Part model, mm, in its own coordinate system. A direction names the side the tool comes from. Coordinates: 2 decimals unless noted, no trailing zeros. Order: outer loops, then holes, each group sorted by start corner. A loop starts at its lowest first (then second) coordinate and runs counter-clockwise, first axis right, second up.
```python
from build123d import *
from build123d.topology import SkipClean

# Parameters (mm, degrees)
CROQUIS1_R                                           = 11.75
SALIENTE_EXTRUIR1_DEPTH                              = 5
REFRENTADO_PARA_TORNILLO_CON_CABEZA_PLAN_D           = 2
REFRENTADO_PARA_TORNILLO_CON_CABEZA_PLAN_CBORE_D     = 4
REFRENTADO_PARA_TORNILLO_CON_CABEZA_PLAN_CBORE_DEPTH = 2.5
CROQUIS6_R                                           = 4.25
CORTAR_EXTRUIR1_DEPTH                                = 1.9
CROQUIS7_R                                           = 5.75
SALIENTE_EXTRUIR2_DEPTH                              = 15
CROQUIS8_R                                           = 5.75
SALIENTE_EXTRUIR3_DEPTH                              = 10
CROQUIS9_R                                           = 3.55
CORTAR_EXTRUIR2_DEPTH                                = 20
SALIENTE_EXTRUIR4_DEPTH                              = 10
CORTAR_EXTRUIR3_DEPTH                                = 3
MATRIZC1_COUNT                                       = 4


with BuildPart() as part:
    # Croquis1 → Saliente-Extruir1 (new body)
    with BuildSketch(Plane.XY):
        Circle(CROQUIS1_R)
    extrude(amount=SALIENTE_EXTRUIR1_DEPTH)

    # Refrentado para tornillo con cabeza plana de M21 (through all)
    with Locations(Plane(origin=(0, 8, 5), x_dir=(1, 0, 0), z_dir=(0, 0, 1))):
        with Locations((0, 0), (7.999986777, -7.985454569), (0, -16), (-8, -8)):
            CounterBoreHole(REFRENTADO_PARA_TORNILLO_CON_CABEZA_PLAN_D / 2, REFRENTADO_PARA_TORNILLO_CON_CABEZA_PLAN_CBORE_D / 2, REFRENTADO_PARA_TORNILLO_CON_CABEZA_PLAN_CBORE_DEPTH)

    # Croquis6 → Cortar-Extruir1 (cut)
    with BuildSketch(Plane(origin=(0, 0, 0), x_dir=(-1, 0, 0), z_dir=(0, 0, -1))):
        with Locations((0, 0.014473443)):
            Circle(CROQUIS6_R)
    extrude(amount=-CORTAR_EXTRUIR1_DEPTH, mode=Mode.SUBTRACT)

    # Croquis7 → Saliente-Extruir2 (add)
    with BuildSketch(Plane.XY.offset(5)):
        Circle(CROQUIS7_R)
    extrude(amount=SALIENTE_EXTRUIR2_DEPTH)

    # Croquis8 → Saliente-Extruir3 (add)
    with BuildSketch(Plane.XY.offset(20)):
        Circle(CROQUIS8_R)
    extrude(amount=SALIENTE_EXTRUIR3_DEPTH)

    # Croquis9 → Cortar-Extruir2 (cut)
    with BuildSketch(Plane.XY.offset(30)):
        Circle(CROQUIS9_R)
    extrude(amount=-CORTAR_EXTRUIR2_DEPTH, mode=Mode.SUBTRACT)

    # Croquis10 → Saliente-Extruir4 (add)
    with SkipClean():  # the faces are left unmerged after this step: merging them gives an invalid solid
        with BuildSketch(Plane.XY.offset(5)):
            with BuildLine():
                Line((-7.342883246, 5.221562902), (-9.301185034, 7.17986469))
                ThreePointArc((-9.301185034, 7.17986469), (-8.308504679, 8.308504679), (-7.17986469, 9.301185034))
                Line((-7.17986469, 9.301185034), (-5.221562902, 7.342883246))
                Line((-5.221562902, 7.342883246), (-2.864419445, 4.985739789))
                ThreePointArc((-2.864419445, 4.985739789), (-4.065863992, 4.065863992), (-4.985739789, 2.864419445))
                Line((-4.985739789, 2.864419445), (-7.342883246, 5.221562902))
            make_face()
        saliente_extruir4 = extrude(amount=SALIENTE_EXTRUIR4_DEPTH)

    # Croquis11 → Cortar-Extruir3 (cut)
    with BuildSketch(Plane(origin=(-1.060660172, -1.060660172, 0), x_dir=(0, 0, 1), z_dir=(-0.7071067811865472, -0.7071067811865478, 0))):
        Polygon((15, 5.550900828), (15, 11.784165538), (5, 11.780723295), (5, 11.653862021), align=None)
    cortar_extruir3 = extrude(amount=-CORTAR_EXTRUIR3_DEPTH, mode=Mode.SUBTRACT)

    # MatrizC1: Saliente-Extruir4, Cortar-Extruir3 ×4 about axis
    with SkipClean():  # the faces are left unmerged after this step: merging them gives an invalid solid
        matrizc1_axis = Axis((0, 0, 0), (0, 0, 1))
        add([saliente_extruir4.rotate(matrizc1_axis, i * 360 / MATRIZC1_COUNT) for i in range(1, MATRIZC1_COUNT)])
        add([cortar_extruir3.rotate(matrizc1_axis, i * 360 / MATRIZC1_COUNT) for i in range(1, MATRIZC1_COUNT)], mode=Mode.SUBTRACT)


solid = part.part
```
(1) Drop flat-ended pins along their axis: pin 1 (4 mm diameter, centred on x = -7, y = -9, fed in from +Z); pin 2 (3 mm diameter, centred on x = -9, y = -1, fed in from +Z); pin 3 (4 mm diameter, centred on y = 9, z = 4.5, fed in from +X). Give the stop position or say it passes through.
(2) Slice it at C-C, the plane z = 10.5. Give the cut face in (x, y).
(3) Slice it at A-A, the plane x = 0. State how many separate pieces and enclosed holes the cut face has, then the cut area to 3 significant figures.
(4) Probe line 1 (Y direction, x = 0, z = 1.3); line 2 (Y direction, x = 0, z = 4.1); line 3 (Y direction, x = -0.5, z = 3.5). List the from-to ranges inside material, lowest first.
(5) Slice it at B-B, the plane y = 8. Give the cut face in (x, z).
(6) Tool access for faces 1 (the face through (-6.21, 4.09, 7.71)), 2 (the face through (6, 0, 4)), 3 (the face through (4.51, -6.63, 8.82)): list every direction of +Z, -Z, +X, -X, +Y, -Y with a clear straight run to the whole face (end or side of a thin tool).
Here are the results:
1. pin 1: stops at z = 8.83
1. pin 2: stops at z = 5
1. pin 3: stops at x = 9.44
2. outline: (-6.93, -4.81) - (-4.81, -6.93) - (-2.86, -4.99) arc R5.75 ccw to (2.86, -4.99) - (4.81, -6.93) - (6.93, -4.81) - (4.99, -2.86) arc R5.75 ccw to (4.99, 2.86) - (6.93, 4.81) - (4.81, 6.93) - (2.86, 4.99) arc R5.75 ccw to (-2.86, 4.99) - (-4.81, 6.93) - (-6.93, 4.81) - (-4.99, 2.86) arc R5.75 ccw to (-4.99, -2.86) - close; hole circle Ø7.1 at (0, 0)
3. separate pieces: 3
3. enclosed holes: 0
3. area: 217 mm2
4. line 1: y = -11.75 to -9, -7 to -4.24, 4.26 to 7, 9 to 11.75
4. line 2: y = -11.75 to -10, -6 to 6, 10 to 11.75
4. line 3: y = -11.74 to -9.94, -6.06 to 6.06, 9.94 to 11.74
5. outline: (-8.61, 0) - (-1, 0) - (-1, 2.5) - (-2, 2.5) - (-2, 5) - (-5.88, 5) - (-5.88, 8.02) - (-8.48, 5) - (-8.61, 5) - close; (1, 0) - (8.61, 0) - (8.61, 5) - (8.48, 5) - (5.88, 8.02) - (5.88, 5) - (2, 5) - (2, 2.5) - (1, 2.5) - close
6. face 1: +Z, -X
6. face 2: +Z
6. face 3: +Z, -Y
